Source: CAD feature listing. Evaluate the final solid. Frame: model axes, mm. A direction names the side the tool comes from. Coordinates: 2 decimals unless noted, no trailing zeros. Write each loop counter-clockwise with the first axis right and the second up, starting at its lowest first coordinate (ties: lowest second). Pieces come first, ordered by that corner, then holes. Notation, with made-up numbers: (-14.5, 72) -> (1.5, 72) arc R25 ccw to (1.5, 92) -> close; hole circle Ø11 at (32.5, 75). An arc over 180 degrees is marked (long way). One line per item, written item: value. Start each with the question number.
1. Mould query, pull axis X, two halves, no side actions, for faces 5 (the flat face through (-53, 2.7, -42)), 6 (the cylindrical face through (-51.14, -0.18, -2.4)), 7 (the flat face through (-55, 0, -29)). Classes: released by +X, released by -X, zero draft, split by the parting line, or undercut.
2. Section query B-B, the plane y = 10. Output: boundary loops of the cut face in (x, z), and give its area (3 significant figures).
3. Line query: line 1 (X direction, y = 6.75, z = -16.5); line 2 (Z direction, x = -7, y = -3.25). Output: solid intervals per line, ascending.
4. Section query D-D, the plane y = 4.25. Output: boundary loops of the cut face in (x, z), and give its area (3 significant figures).
5. Section query A-A, the plane x = 20.5. Output: boundary loops of the cut face in (y, z), and give its area (3 significant figures).
6. Section query C-C, the plane z = -11. Output: boundary loops of the cut face in (x, y), and give its area (3 significant figures).
7. First-contact query: P1, Ø8, axis at x = -36.5, y = 1.5, coming from the -Z side; P2, Ø2, axis at y = 0, z = -51.5, coming from the +X side. Flat tips, straight axial feed; report the tip coordinate or a pass-through.
8. Access query for faces 1 (the flat face through (0, -12.5, -1)), 2 (the flat face through (-53.479, -1.369, -43.827)), 3 (the cylindrical face through (53.52, 0.38, -52.69)), 4 (the flat face through (-1, 0, -1.5)). Directions: +Z, -Z, +X, -X, +Y, -Y. A direction counts if a zero-diameter tool reaches every point of the face in a straight line with its end or side. Return the directions, or none.
from build123d import *

# Parameters (mm, degrees)
T_LE_START                            = -1.5
T_LE_DE_BASE_PLI_E2_OUTLINE_W         = 104
T_LE_DE_BASE_PLI_E2_OUTLINE_H         = 25
T_LE_DE_BASE_PLI_E2_DEPTH             = 3
T_LE_PLI_E_SUR_AR_TE1_STRIP_W         = 18
T_LE_PLI_E_SUR_AR_TE1_STRIP_H         = 3
T_LE_PLI_E_SUR_AR_TE1_STRIP_CUT_DEPTH = 25
T_LE_PLI_E_SUR_AR_TE1_DEPTH           = 25
T_LE_PLI_E_SUR_AR_TE2_STRIP_W         = 18
T_LE_PLI_E_SUR_AR_TE2_STRIP_H         = 3
T_LE_PLI_E_SUR_AR_TE2_STRIP_CUT_DEPTH = 25
T_LE_PLI_E_SUR_AR_TE2_DEPTH           = 25
ENL_V_MAT_EXTRU_1_REACH               = 72.924
ESQUISSE20_R                          = 1.75
PATTE1_DEPTH                          = 3
PATTE2_START                          = -3
PATTE2_DEPTH                          = 3
ENL_V_MAT_EXTRU_2_REACH               = 125.176
ESQUISSE27_R                          = 1.25
ENL_V_MAT_EXTRU_3_REACH               = 122.504
ENL_V_MAT_EXTRU_4_REACH               = 125.176
ESQUISSE29_R                          = 1.7


# Read off the part's stored shape, not the designer's step: Tôle de base pliée2
# Sheet-metal steps are written as plain solids
with BuildPart() as part:
    # Tôle de base pliée2 outline → Tôle de base pliée2 (new body)
    with BuildSketch(Plane.XY.offset(T_LE_START)):
        Rectangle(T_LE_DE_BASE_PLI_E2_OUTLINE_W, T_LE_DE_BASE_PLI_E2_OUTLINE_H)
    extrude(amount=T_LE_DE_BASE_PLI_E2_DEPTH)

    # Tôle pliée sur arête1 strip (across the edge) → Tôle pliée sur arête1 strip cut (cut)
    with BuildSketch(Plane(origin=(52, 12.5, -1.5), x_dir=(-1, 0, 0), z_dir=(0, -1, 0))):
        with Locations((-6, -1.5)):
            Rectangle(T_LE_PLI_E_SUR_AR_TE1_STRIP_W, T_LE_PLI_E_SUR_AR_TE1_STRIP_H)
    extrude(amount=T_LE_PLI_E_SUR_AR_TE1_STRIP_CUT_DEPTH, mode=Mode.SUBTRACT)

    # Tôle pliée sur arête1 section (across the edge) → Tôle pliée sur arête1 (add)
    with BuildSketch(Plane(origin=(52, 12.5, -1.5), x_dir=(-1, 0, 0), z_dir=(0, -1, 0))):
        with BuildLine():
            Line((-3, 3), (-3, 40))
            Line((-3, 40), (0, 40))
            Line((0, 40), (0, 3))
            ThreePointArc((0, 3), (0.878679656, 0.878679656), (3, 0))
            Line((3, 0), (3, -3))
            ThreePointArc((3, -3), (-1.242640687, -1.242640687), (-3, 3))
        make_face()
    extrude(amount=T_LE_PLI_E_SUR_AR_TE1_DEPTH)

    # Tôle pliée sur arête2 strip (across the edge) → Tôle pliée sur arête2 strip cut (cut)
    with BuildSketch(Plane(origin=(-52, -12.5, -1.5), x_dir=(1, 0, 0), z_dir=(0, 1, 0))):
        with Locations((-6, -1.5)):
            Rectangle(T_LE_PLI_E_SUR_AR_TE2_STRIP_W, T_LE_PLI_E_SUR_AR_TE2_STRIP_H)
    extrude(amount=T_LE_PLI_E_SUR_AR_TE2_STRIP_CUT_DEPTH, mode=Mode.SUBTRACT)

    # Tôle pliée sur arête2 section (across the edge) → Tôle pliée sur arête2 (add)
    with BuildSketch(Plane(origin=(-52, -12.5, -1.5), x_dir=(1, 0, 0), z_dir=(0, 1, 0))):
        with BuildLine():
            Line((-3, 3), (-3, 40))
            Line((-3, 40), (0, 40))
            Line((0, 40), (0, 3))
            ThreePointArc((0, 3), (0.878679656, 0.878679656), (3, 0))
            Line((3, 0), (3, -3))
            ThreePointArc((3, -3), (-1.242640687, -1.242640687), (-3, 3))
        make_face()
    extrude(amount=T_LE_PLI_E_SUR_AR_TE2_DEPTH)

    # Esquisse20 → Enlèv. mat.-Extru.1 (cut, up to next)
    with BuildSketch(Plane.XY.offset(1.5), mode=Mode.PRIVATE) as enl_v_mat_extru_1_sk1:
        with Locations((-7.5, 0)):
            Circle(ESQUISSE20_R)
    enl_v_mat_extru_1_tool1 = extrude(enl_v_mat_extru_1_sk1.sketch, amount=-ENL_V_MAT_EXTRU_1_REACH, mode=Mode.PRIVATE) & part.part
    # Esquisse20 → Enlèv. mat.-Extru.1 (cut, up to next)
    with BuildSketch(Plane.XY.offset(1.5), mode=Mode.PRIVATE) as enl_v_mat_extru_1_sk2:
        with Locations((20.5, 0)):
            Circle(ESQUISSE20_R)
    enl_v_mat_extru_1_tool2 = extrude(enl_v_mat_extru_1_sk2.sketch, amount=-ENL_V_MAT_EXTRU_1_REACH, mode=Mode.PRIVATE) & part.part
    add(enl_v_mat_extru_1_tool1.solids().sort_by_distance((-7.5, 0, 1.5))[0], mode=Mode.SUBTRACT)
    add(enl_v_mat_extru_1_tool2.solids().sort_by_distance((20.5, 0, 1.5))[0], mode=Mode.SUBTRACT)

    # Esquisse21 → Patte1 (add)
    with BuildSketch(Plane.ZY.offset(55)):
        with BuildLine():
            Line((-41.5, 12.5), (-41.5, -12.5))
            ThreePointArc((-41.5, -12.5), (-54, 0), (-41.5, 12.5))
        make_face()
    extrude(amount=-PATTE1_DEPTH)

    # Esquisse24 → Patte2 (add)
    with BuildSketch(Plane(origin=(55, 0, 0), x_dir=(0, 0, -1), z_dir=(1, 0, 0)).offset(PATTE2_START)):
        with BuildLine():
            Line((41.5, 12.5), (41.5, -12.5))
            ThreePointArc((41.5, -12.5), (54, 0), (41.5, 12.5))
        make_face()
    extrude(amount=PATTE2_DEPTH)

    # Esquisse27 → Enlèv. mat.-Extru.2 (cut, up to next)
    with BuildSketch(Plane(origin=(55, 0, 0), x_dir=(0, 0, -1), z_dir=(1, 0, 0)), mode=Mode.PRIVATE) as enl_v_mat_extru_2_sk1:
        with Locations((51.5, 0)):
            Circle(ESQUISSE27_R)
    enl_v_mat_extru_2_tool1 = extrude(enl_v_mat_extru_2_sk1.sketch, amount=-ENL_V_MAT_EXTRU_2_REACH, mode=Mode.PRIVATE) & part.part
    # Esquisse27 → Enlèv. mat.-Extru.2 (cut, up to next)
    with BuildSketch(Plane(origin=(55, 0, 0), x_dir=(0, 0, -1), z_dir=(1, 0, 0)), mode=Mode.PRIVATE) as enl_v_mat_extru_2_sk2:
        with Locations((41.5, -10)):
            Circle(ESQUISSE27_R)
    enl_v_mat_extru_2_tool2 = extrude(enl_v_mat_extru_2_sk2.sketch, amount=-ENL_V_MAT_EXTRU_2_REACH, mode=Mode.PRIVATE) & part.part
    # Esquisse27 → Enlèv. mat.-Extru.2 (cut, up to next)
    with BuildSketch(Plane(origin=(55, 0, 0), x_dir=(0, 0, -1), z_dir=(1, 0, 0)), mode=Mode.PRIVATE) as enl_v_mat_extru_2_sk3:
        with Locations((31.5, 0)):
            Circle(ESQUISSE27_R)
    enl_v_mat_extru_2_tool3 = extrude(enl_v_mat_extru_2_sk3.sketch, amount=-ENL_V_MAT_EXTRU_2_REACH, mode=Mode.PRIVATE) & part.part
    # Esquisse27 → Enlèv. mat.-Extru.2 (cut, up to next)
    with BuildSketch(Plane(origin=(55, 0, 0), x_dir=(0, 0, -1), z_dir=(1, 0, 0)), mode=Mode.PRIVATE) as enl_v_mat_extru_2_sk4:
        with Locations((41.5, 10)):
            Circle(ESQUISSE27_R)
    enl_v_mat_extru_2_tool4 = extrude(enl_v_mat_extru_2_sk4.sketch, amount=-ENL_V_MAT_EXTRU_2_REACH, mode=Mode.PRIVATE) & part.part
    add(enl_v_mat_extru_2_tool1.solids().sort_by_distance((55, 0, -51.5))[0], mode=Mode.SUBTRACT)
    add(enl_v_mat_extru_2_tool2.solids().sort_by_distance((55, -10, -41.5))[0], mode=Mode.SUBTRACT)
    add(enl_v_mat_extru_2_tool3.solids().sort_by_distance((55, 0, -31.5))[0], mode=Mode.SUBTRACT)
    add(enl_v_mat_extru_2_tool4.solids().sort_by_distance((55, 10, -41.5))[0], mode=Mode.SUBTRACT)

    # Esquisse28 → Enlèv. mat.-Extru.3 (cut, up to next)
    with BuildSketch(Plane(origin=(-52, 0, 0), x_dir=(0, 0, -1), z_dir=(1, 0, 0)), mode=Mode.PRIVATE) as enl_v_mat_extru_3_sk1:
        Polygon((43.058845727, -2.7), (44.617691454, 0), (43.058845727, 2.7), (39.941154273, 2.7), (38.382308546, 0), (39.941154273, -2.7), align=None)
    enl_v_mat_extru_3_tool1 = extrude(enl_v_mat_extru_3_sk1.sketch, amount=-ENL_V_MAT_EXTRU_3_REACH, mode=Mode.PRIVATE) & part.part
    add(enl_v_mat_extru_3_tool1.solids().sort_by_distance((-52, 0, -41.5))[0], mode=Mode.SUBTRACT)

    # Esquisse29 → Enlèv. mat.-Extru.4 (cut, up to next)
    with BuildSketch(Plane.ZY.offset(55), mode=Mode.PRIVATE) as enl_v_mat_extru_4_sk1:
        with Locations((-50.25, 0)):
            Circle(ESQUISSE29_R)
    enl_v_mat_extru_4_tool1 = extrude(enl_v_mat_extru_4_sk1.sketch, amount=-ENL_V_MAT_EXTRU_4_REACH, mode=Mode.PRIVATE) & part.part
    # Esquisse29 → Enlèv. mat.-Extru.4 (cut, up to next)
    with BuildSketch(Plane.ZY.offset(55), mode=Mode.PRIVATE) as enl_v_mat_extru_4_sk2:
        with Locations((-32.75, 0)):
            Circle(ESQUISSE29_R)
    enl_v_mat_extru_4_tool2 = extrude(enl_v_mat_extru_4_sk2.sketch, amount=-ENL_V_MAT_EXTRU_4_REACH, mode=Mode.PRIVATE) & part.part
    add(enl_v_mat_extru_4_tool1.solids().sort_by_distance((-55, 0, -50.25))[0], mode=Mode.SUBTRACT)
    add(enl_v_mat_extru_4_tool2.solids().sort_by_distance((-55, 0, -32.75))[0], mode=Mode.SUBTRACT)


solid = part.part
Computed values:
1. face 5: zero draft
1. face 6: undercut
1. face 7: released by -X
2. outline: (-55, -49) -> (-52, -49) -> (-52, -4.5) arc R3 cw to (-49, -1.5) -> (49, -1.5) arc R3 cw to (52, -4.5) -> (52, -40.25) -> (55, -40.25) -> (55, -4.5) arc R6 ccw to (49, 1.5) -> (-49, 1.5) arc R6 ccw to (-55, -4.5) -> close; (52, -49) -> (55, -49) -> (55, -42.75) -> (52, -42.75) -> close
2. area: 596 mm²
3. line 1: x = -55 to -52, 52 to 55
3. line 2: z = -1.5 to 1.5
4. outline: (-55, -53.26) -> (-52, -53.26) -> (-52, -4.5) arc R3 cw to (-49, -1.5) -> (49, -1.5) arc R3 cw to (52, -4.5) -> (52, -53.26) -> (55, -53.26) -> (55, -4.5) arc R6 ccw to (49, 1.5) -> (-49, 1.5) arc R6 ccw to (-55, -4.5) -> close
4. area: 629 mm²
5. outline: (-12.5, -1.5) -> (-1.75, -1.5) -> (-1.75, 1.5) -> (-12.5, 1.5) -> close; (1.75, -1.5) -> (12.5, -1.5) -> (12.5, 1.5) -> (1.75, 1.5) -> close
5. area: 64.5 mm²
6. outline: (-55, -12.5) -> (-52, -12.5) -> (-52, 12.5) -> (-55, 12.5) -> close; (52, -12.5) -> (55, -12.5) -> (55, 12.5) -> (52, 12.5) -> close
6. area: 150 mm²
7. P1: stops at z = -1.5
7. P2: stops at x = -52
8. face 1: +Z, -Z, +X, -X, -Y
8. face 2: -X
8. face 3: +X
8. face 4: -Z, +Y, -Y
